Autodesk Inventor part; units mm, degrees
ref_plane "YZ Plane" through (0, 0, 0) normal (1, 0, 0) x (0, 1, 0)
ref_plane "XZ Plane" through (0, 0, 0) normal (0, 1, 0) x (-1, 0, 0)
ref_plane "XY Plane" through (0, 0, 0) normal (0, 0, 1) x (1, 0, 0)
sketch "main" plane through (0, 0, 0) normal (0, 0, 1) x (1, 0, 0)
  circle A0 centre (70.448, 399.2567) radius 2.1844
  circle A1 centre (95.848, 399.2567) radius 2.1844
  circle A2 centre (83.148, 421.4817) radius 9.398
  arc A3 (95.848, 392.9067) -> (102.1377, 400.1294) centre (95.848, 399.2567) ccw
  arc A4 (64.1582, 400.1294) -> (70.448, 392.9067) centre (70.448, 399.2567) ccw
  line L0 (95.848, 392.9067) -> (70.448, 392.9067)
  arc A5 (98.8723, 423.6635) -> (67.4236, 423.6635) centre (83.148, 421.4817) ccw
  line L1 (102.1377, 400.1294) -> (98.8723, 423.6635)
  line L2 (67.4236, 423.6635) -> (64.1582, 400.1294)
  point P0 (83.148, 405.9327)
  dimension "d0" = 18.796
  dimension "d1" = 12.7
  dimension "d2" = 12.7
sketch "Sketch1" plane through (0, 0, 0) normal (0, 0, 1) x (1, 0, 0)
  circle A0 centre (2.5908, 29.8069) radius 2.0955
  circle A1 centre (22.8092, 29.8069) radius 2.0955
  circle A2 centre (0, 0) radius 2.1844
  circle A3 centre (25.4, 0) radius 2.1844
  circle A4 centre (12.7, 22.225) radius 9.398
  arc A5 (25.4, -6.35) -> (31.6897, 0.8727) centre (25.4, 0) ccw
  arc A6 (-6.2897, 0.8727) -> (0, -6.35) centre (0, 0) ccw
  line L0 (25.4, -6.35) -> (0, -6.35)
  arc A7 (28.4244, 24.4068) -> (-3.0244, 24.4068) centre (12.7, 22.225) ccw
  line L1 (31.6897, 0.8727) -> (28.4244, 24.4068)
  line L2 (-3.0244, 24.4068) -> (-6.2897, 0.8727)
  dimension "d5" = 4.191
  dimension "d6" = 4.191
extrude "Extrusion1" add sketch "Sketch1" along normal blind 1.5875
properties part number "resevoir_mount" material "Acetal Resin, White"
Build history of the part. All positions in model axes, mm. Coordinates: 2 decimals unless noted, no trailing zeros. Order: outer loops, then holes, each group sorted by start corner. A loop starts at its lowest first (then second) coordinate and runs counter-clockwise, first axis right, second up. Notation, with made-up numbers: (29.25, 15.25) - (84.25, 15.25) arc R29 ccw to (84.25, 37.25) - close; hole circle Ø7 at (82, 31). An arc over 180 degrees is marked (long way). Put each result on its own line as item: value.
1. Probe line 1 along Y through (x, z) = (24.5, 1.15); line 2 along Y through (x, z) = (0, 1.05). List the from-to ranges inside material, lowest first. Write a range as [from, to].
Answer sheet:
line 1: y = [-6.35, -1.99], [1.99, 28.57], [31.04, 32.84]
line 2: y = [-6.35, -2.18], [2.18, 31.75]
2. Pull direction Y, two halves, no side cores. Call faces 1 (the face through (13, -6.35, 1)), 2 (the face through (22.35, 31.85, 0.78)), 3 (the face through (30.08, 12.48, 0.78)), 4 (the face through (12, 11, 1.588)): pulls with the +Y half, pulls with the -Y half, needs draft (parallel to the pull), parting line crosses it, or undercut.
Answer sheet:
face 1: pulls with the -Y half
face 2: undercut
face 3: pulls with the +Y half
face 4: needs draft
3. Saw through at A-A (y = 0). Write the cut outline in (x, z).
Answer sheet:
outline: (-6.35, 0) - (-2.18, 0) - (-2.18, 1.59) - (-6.35, 1.59) - close; (2.18, 0) - (23.22, 0) - (23.22, 1.59) - (2.18, 1.59) - close; (27.58, 0) - (31.75, 0) - (31.75, 1.59) - (27.58, 1.59) - close
4. Saw through at C-C (y = 16). Write the cut outline in (x, z).
Answer sheet:
outline: (-4.19, 0) - (5.66, 0) - (5.66, 1.59) - (-4.19, 1.59) - close; (19.74, 0) - (29.59, 0) - (29.59, 1.59) - (19.74, 1.59) - close
5. Saw through at B-B (x = 12.7). Write the cut outline in (y, z), and give its area (3 significant figures).
Answer sheet:
outline: (-6.35, 0) - (12.83, 0) - (12.83, 1.59) - (-6.35, 1.59) - close; (31.62, 0) - (38.1, 0) - (38.1, 1.59) - (31.62, 1.59) - close
area: 40.7 mm^2
6. Saw through at D-D (z = 0.4). Give the number of separate pieces and of enclosed holes in the cut face, and give its area (3 significant figures).
Answer sheet:
separate pieces: 1
enclosed holes: 5
area: 1,070 mm^2
7. Drop a flat-ended pin along its axis: P1, Ø3.5, axis at x = 2.59, y = 29.81, coming from the +Z side. Give the stop position or say it passes through.
Answer sheet:
P1: passes through
